Source: CAD feature listing. Evaluate the final solid. Frame: model axes, mm. A direction names the side the tool comes from. Round coordinates to 2 decimals unless told otherwise and drop trailing zeros. Order: outer loops, then holes, each group sorted by start corner. A loop starts at its lowest first (then second) coordinate and runs counter-clockwise, first axis right, second up. Notation, with made-up numbers: M 21,27.5 L 80,27.5 A5 ccw 80,36.5 Z; hole C 57.25,32.25 d9. An arc over 180 degrees is marked long. Answer as CSV lines item,"result". Start each with the question number.
Item 1: Section query C-C on y = 0. Return the cut outline in (x, z) (3 decimals).
Item 2: Section query B-B on z = 1.25. State how many separate pieces and enclosed holes the cut face has, plus the area to 3 significant figures.
Item 3: Line query: line 1 (Y direction, x = 0, z = 4.25); line 2 (X direction, y = -1, z = 2.5) (3 decimals); line 3 (Y direction, x = -28, z = 2.5). Output: solid intervals per line, ascending. Write a range as [from, to].
Item 4: Section query A-A on x = 0. Return the cut outline in (y, z).
Item 5: Set-up query: faces 1 (the face through (63, 20, 3)), 2 (the face through (10, 23, 3)), 3 (the face through (-20, -20, 3)), 4 (the face through (50, -23, 3)). Return all of +Z, -Z, +X, -X, +Y, -Y with unobstructed straight access to the full face (end or side cutting, diameter ignored); none if empty.
Item 6: First-contact query: P1, Ø13, axis at x = 60.675, y = -4.35, coming from the +Z side; P2, Ø3, axis at y = -22.5, z = 2.5, coming from the +X side; P3, Ø3, axis at x = 17.5, z = 2.5, coming from the +Y side; P4, Ø1.9, axis at y = 23.5, z = 2, coming from the -X side. Flat tips, straight axial feed; report the tip coordinate or a pass-through.
Item 7: Pull-direction query (X, two-part tool) for faces 5 (the face through (-10, -23, 3)), 6 (the face through (63, -20, 3)), 7 (the face through (76.325, 0, 3)); classes: +X half, -X half, draft (parallel to the pull), parting line (faces both ways), or undercut.
from build123d import *

# Parameters (mm, degrees)
ESQUISSE1_W             = 165.35
ESQUISSE1_H             = 52.7
BOSS_EXTRU_1_DEPTH      = 6.35
ESQUISSE5_W             = 20
ESQUISSE5_H             = 6.35
ESQUISSE5_W_2           = 26.325
ENL_V_MAT_EXTRU_2_DEPTH = 88.004601171
ESQUISSE7_W             = 6.35
ESQUISSE7_H             = 52.7
ENL_V_MAT_EXTRU_4_DEPTH = 88.004601171
ESQUISSE6_R             = 8
ENL_V_MAT_EXTRU_3_DEPTH = 81.994756775


with BuildPart() as part:
    # Esquisse1 → Boss.-Extru.1 (new body)
    with BuildSketch(Plane.XY):
        Rectangle(ESQUISSE1_W, ESQUISSE1_H)
    extrude(amount=BOSS_EXTRU_1_DEPTH)

    # Esquisse5 → Enlèv. mat.-Extru.2 (cut, through all)
    with BuildSketch(Plane.XY.offset(6.35)):
        with Locations((-20, -23.175)):
            Rectangle(ESQUISSE5_W, ESQUISSE5_H)
        with Locations((20, -23.175)):
            Rectangle(ESQUISSE5_W, ESQUISSE5_H)
        with Locations((63.1625, -23.175)):
            Rectangle(ESQUISSE5_W_2, ESQUISSE5_H)
        with Locations((-63.1625, -23.175)):
            Rectangle(ESQUISSE5_W_2, ESQUISSE5_H)
    enl_v_mat_extru_2 = extrude(amount=-ENL_V_MAT_EXTRU_2_DEPTH, mode=Mode.SUBTRACT)

    # Symétrie2: Enlèv. mat.-Extru.2 across plane
    add(enl_v_mat_extru_2.mirror(Plane.ZX), mode=Mode.SUBTRACT)

    # Esquisse7 → Enlèv. mat.-Extru.4 (cut, through all)
    with BuildSketch(Plane.XY.offset(6.35)):
        with Locations((-79.5, 0)):
            Rectangle(ESQUISSE7_W, ESQUISSE7_H)
        with Locations((79.5, 0)):
            Rectangle(ESQUISSE7_W, ESQUISSE7_H)
    extrude(amount=-ENL_V_MAT_EXTRU_4_DEPTH, mode=Mode.SUBTRACT)

    # Esquisse6 → Enlèv. mat.-Extru.3 (cut, through all)
    with BuildSketch(Plane.XY.offset(6.35)):
        Circle(ESQUISSE6_R)
        with Locations((60.675, -4.35)):
            Circle(ESQUISSE6_R)
    extrude(amount=-ENL_V_MAT_EXTRU_3_DEPTH, mode=Mode.SUBTRACT)


solid = part.part
Results:
1,outline,"M -76.325,0 L -8,0 L -8,6.35 L -76.325,6.35 Z; M 8,0 L 53.961,0 L 53.961,6.35 L 8,6.35 Z; M 67.389,0 L 76.325,0 L 76.325,6.35 L 67.389,6.35 Z"
2,separate pieces,"1"
2,enclosed holes,"2"
2,area,"6,470 mm^2"
3,line 1,"[-26.35, -8], [8, 26.35]"
3,line 2,"[-76.325, -7.937], [7.937, 53.41], [67.94, 76.325]"
3,line 3,"[-20, 20]"
4,outline,"M -26.35,0 L -8,0 L -8,6.35 L -26.35,6.35 Z; M 8,0 L 26.35,0 L 26.35,6.35 L 8,6.35 Z"
5,face 1,"+Z, -Z, +X, +Y"
5,face 2,"+Z, -Z, +Y"
5,face 3,"+Z, -Z, -Y"
5,face 4,"+Z, -Z, +X, -Y"
6,P1,"through"
6,P2,"x = 50"
6,P3,"y = 20"
6,P4,"x = -50"
7,face 5,"undercut"
7,face 6,"draft"
7,face 7,"+X half"
